Could you check a few things on this model? Use its own coordinates, in mm. A direction names the side the tool comes from. Round coordinates to 2 decimals unless told otherwise and drop trailing zeros. Loops run counter-clockwise (first coordinate to the right, second up) from the corner with the lowest first, then second, coordinate; pieces in that order, holes last. Notation, with made-up numbers: (-39.75, -11) -> (-0.75, -11) arc R30 ccw to (-0.75, 16) -> close; hole circle Ø5 at (-4.75, -2.75). An arc over 180 degrees is marked (long way). One line per item, written item: value.
```python
from build123d import *

# Parameters (mm, degrees)
F2_R     = 2.6
F3_DEPTH = 2.35
F4_R     = 8.635865
F4_R_2   = 6.173243
F5_DEPTH = 2


with BuildPart() as f1:
    # F0 (on Front) → F1 (revolve)
    with BuildSketch(Plane.XZ):
        Polygon((-3.9, 7.43), (-11, 7.43), (-11, 2.35), (-21.95, 2.35), (-21.95, 0), (-11, 0), (-11, -20.07), (0, -20.07), (0, 16.43), (-3.9, 16.43), align=None)
    revolve(axis=Axis((0, 0, -1.82), (0, 0, -1)))

    # F2 (on face) → F3 (cut, through all)
    with BuildSketch(Plane.XY.offset(2.35)):
        with Locations((0, 17.45)):
            Circle(F2_R)
        with Locations((15.112143, -8.725)):
            Circle(F2_R)
        with Locations((-15.112143, -8.725)):
            Circle(F2_R)
    extrude(amount=-F3_DEPTH, mode=Mode.SUBTRACT)

    # F4 (on face) → F5 (cut)
    with BuildSketch(Plane.XY.offset(7.43)):
        Circle(F4_R)
        Circle(F4_R_2, mode=Mode.SUBTRACT)
    extrude(amount=-F5_DEPTH, mode=Mode.SUBTRACT)


solid = f1.part
```
Item 1: I need wall thicknesses on line 1 (Y direction, x = 0, z = 6); line 2 (Y direction, x = 0, z = 1.4); line 3 (Z direction, x = 10, y = -2). Which ranges of each line are inside material? Lowest first, please. Write a range as from..to.
Output:
line 1: y = -11..-8.64, -6.17..6.17, 8.64..11
line 2: y = -21.95..14.85, 20.05..21.95
line 3: z = -20.07..7.43
Item 2: If we mould it in two halves opening along X, with no side actions, what happens to faces 1 (the face through (2.38, -10.74, 4.85)), 2 (the face through (-0.56, 14.91, 1.19)), 3 (the face through (1, -4, 7.43))? For each: released by +X, released by -X, zero draft, split by the parting line, or undercut.
Output:
face 1: split by the parting line
face 2: undercut
face 3: zero draft
Item 3: Will these pins go through, and if not, where does the flat tip stop? pin 1 Ø4.5 at (x, y) = (15.11, -8.72) entering from -Z; pin 2 Ø3 at (x, z) = (12, 3) entering from -Y; pin 3 Ø7 at (x, y) = (0, 17.45) entering from -Z; pin 4 Ø5 at (y, z) = (12, -8.5) entering from +X.
Output:
pin 1: passes through
pin 2: stops at y = -19.19
pin 3: stops at z = 0
pin 4: stops at x = 5.55
Item 4: If we section it at A-A on x = 0: List the corners of the cut face in (y, z) for me.
Output:
outline: (-21.95, 0) -> (-11, 0) -> (-11, -20.07) -> (11, -20.07) -> (11, 0) -> (14.85, 0) -> (14.85, 2.35) -> (11, 2.35) -> (11, 7.43) -> (8.64, 7.43) -> (8.64, 5.43) -> (6.17, 5.43) -> (6.17, 7.43) -> (3.9, 7.43) -> (3.9, 16.43) -> (-3.9, 16.43) -> (-3.9, 7.43) -> (-6.17, 7.43) -> (-6.17, 5.43) -> (-8.64, 5.43) -> (-8.64, 7.43) -> (-11, 7.43) -> (-11, 2.35) -> (-21.95, 2.35) -> close; (20.05, 0) -> (21.95, 0) -> (21.95, 2.35) -> (20.05, 2.35) -> close
Item 5: If we section it at C-C on y = 17.45: List the corners of the cut face in (x, z) for me.
Output:
outline: (-13.32, 0) -> (-2.6, 0) -> (-2.6, 2.35) -> (-13.32, 2.35) -> close; (2.6, 0) -> (13.32, 0) -> (13.32, 2.35) -> (2.6, 2.35) -> close
Item 6: If we section it at D-D on y = 0: List the corners of the cut face in (x, z) for me, plus the area to 3 significant figures.
Output:
outline: (-21.95, 0) -> (-11, 0) -> (-11, -20.07) -> (11, -20.07) -> (11, 0) -> (21.95, 0) -> (21.95, 2.35) -> (11, 2.35) -> (11, 7.43) -> (8.64, 7.43) -> (8.64, 5.43) -> (6.17, 5.43) -> (6.17, 7.43) -> (3.9, 7.43) -> (3.9, 16.43) -> (-3.9, 16.43) -> (-3.9, 7.43) -> (-6.17, 7.43) -> (-6.17, 5.43) -> (-8.64, 5.43) -> (-8.64, 7.43) -> (-11, 7.43) -> (-11, 2.35) -> (-21.95, 2.35) -> close
area: 717 mm²
Item 7: If we section it at B-B on y = -10: List the corners of the cut face in (x, z) for me, plus the area to 3 significant figures.
Output:
outline: (-19.54, 0) -> (-17.38, 0) -> (-17.38, 2.35) -> (-19.54, 2.35) -> close; (-12.85, 0) -> (-4.58, 0) -> (-4.58, -20.07) -> (4.58, -20.07) -> (4.58, 0) -> (12.85, 0) -> (12.85, 2.35) -> (4.58, 2.35) -> (4.58, 7.43) -> (-4.58, 7.43) -> (-4.58, 2.35) -> (-12.85, 2.35) -> close; (17.38, 0) -> (19.54, 0) -> (19.54, 2.35) -> (17.38, 2.35) -> close
area: 301 mm²
Item 8: For faces 4 (the face through (0, 0, -20.07)), 5 (the face through (2.38, -10.74, -10.18)), 6 (the face through (-6, 2, 5.43)), which set-ups out of +Z, -Z, +X, -X, +Y, -Y let a thin tool reach every point of the face, with its end or its side?
Output:
face 4: -Z, +X, -X, +Y, -Y
face 5: -Z
face 6: +Z
